Here's the drawing with two shaded views (mm, measured from the low corner). I have some questions. Round coordinates to 2 decimals unless told otherwise and drop trailing zeros. Order: outer loops, then holes, each group sorted by start corner. A loop starts at its lowest first (then second) coordinate and runs counter-clockwise, first axis right, second up. Notation, with made-up numbers: (79.25, 66) -> (104.25, 66) arc R16 cw to (104.25, 72) -> close; hole circle Ø11 at (-39.75, 83). An arc over 180 degrees is marked (long way). Use a Markdown table: item, result. Add a question column.
Q1. If we section it at B-B on z = 25: List the corners of the cut face in (x, y) for me, plus the area to 3 significant figures.
Q2. If we section it at D-D on y = 7.75: List the corners of the cut face in (x, z) for me, plus the area to 3 significant figures.
Q3. If we section it at A-A on x = 25: List the corners of the cut face in (y, z) for me, plus the area to 3 significant figures.
Q4. I'm going to push flat-ended pins straight in: pin 1 Ø2 at (x, y) = (24, 5) entering from -Z; pin 2 Ø8 at (x, z) = (33, 29.5) entering from -Y; pin 3 Ø2 at (y, z) = (7, 32.5) entering from +X. Where does each tip first touch, or does it pass through?
Q5. I need wall thicknesses on line 1 along Z through (x, y) = (24.5, 1.75) (3 decimals); line 2 along Z through (x, y) = (25, 5.55). Which ranges of each line are inside material? Lowest first, please. Write a range as [from, to].
Q6. We'd pull the mould along X, two halves only. Please class the marked faces 1, 2, 3 and 4: +X half, -X half, draft (parallel to the pull), parting line (faces both ways), or undercut.
Q7. If we section it at C-C on y = 2.75: List the corners of the cut face in (x, z) for me.
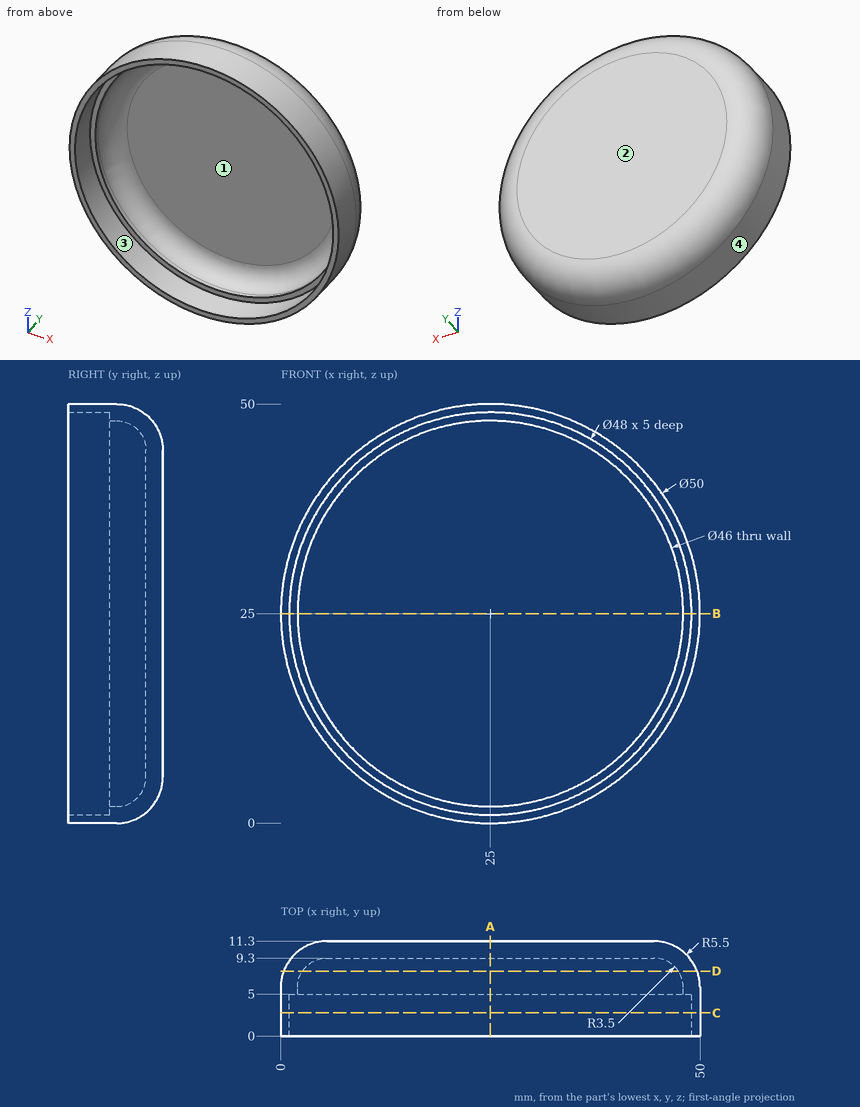
Answer below:
| question | item | result |
|---|---|---|
| 1 | outline | (0, 0) -> (1, 0) -> (1, 5) -> (2, 5) -> (2, 5.8) arc R3.5 cw to (5.5, 9.3) -> (44.5, 9.3) arc R3.5 cw to (48, 5.8) -> (48, 5) -> (49, 5) -> (49, 0) -> (50, 0) -> (50, 5.8) arc R5.5 ccw to (44.5, 11.3) -> (5.5, 11.3) arc R5.5 ccw to (0, 5.8) -> close |
| 1 | area | 119 mm² |
| 2 | outline | circle Ø49.29 at (25, 25); hole circle Ø44.81 at (25, 25) |
| 2 | area | 331 mm² |
| 3 | outline | (0, 0) -> (5.8, 0) arc R5.5 ccw to (11.3, 5.5) -> (11.3, 44.5) arc R5.5 ccw to (5.8, 50) -> (0, 50) -> (0, 49) -> (5, 49) -> (5, 48) -> (5.8, 48) arc R3.5 cw to (9.3, 44.5) -> (9.3, 5.5) arc R3.5 cw to (5.8, 2) -> (5, 2) -> (5, 1) -> (0, 1) -> close |
| 3 | area | 119 mm² |
| 4 | pin 1 | z = 0 |
| 4 | pin 2 | y = 9.3 |
| 4 | pin 3 | x = 49.06 |
| 5 | line 1 | [0.005, 1.005], [48.995, 49.995] |
| 5 | line 2 | [0, 2], [48, 50] |
| 6 | face 1 | undercut |
| 6 | face 2 | draft |
| 6 | face 3 | undercut |
| 6 | face 4 | parting line |
| 7 | outline | circle Ø50 at (25, 25); hole circle Ø48 at (25, 25) |
